```python
from build123d import *

# Parameters (mm, degrees)
F1_DEPTH    = 20
F0_W        = 58.4
F0_H        = 38.4
F2_DEPTH    = 75
F3_T1_DEPTH = 26
F4_R        = 8
F5_W        = 22
F5_H        = 6
F6_DEPTH    = 3


# Not quite as in the source:
# - a fillet or chamfer that OpenCascade refuses, or shapes differently, is made with other operations: its cross-section is extruded or revolved along the edge and cut away or added


with BuildPart() as f1:
    # F0 (on Top) → F1 (new body)
    with BuildSketch(Plane.XY):
        Polygon((20, -35.6130205363), (20, -33.6130205363), (-20, -33.6130205363), (-20, -35.6130205363), (-10, -35.6130205363), (10, -35.6130205363), align=None)
    extrude(amount=F1_DEPTH)

    # F0 (on Top) → F2 (join)
    with BuildSketch(Plane.XY):
        Polygon((20, -33.6130205363), (30, -33.6130205363), (30, 6.3869794637), (-30, 6.3869794637), (-30, -33.6130205363), (-20, -33.6130205363), align=None)
        with Locations((0, -13.6130205363)):
            Rectangle(F0_W, F0_H, mode=Mode.SUBTRACT)
    extrude(amount=F2_DEPTH)

    # F3: fillet of radius 1.2 on 4 edges, made by hand

    # F3_s2 → F3_t1 (cut)
    with BuildSketch(Plane.XY.offset(-3)):
        with BuildLine():
            ThreePointArc((20, -34.4130205363), (19.6485281374, -35.2615486737), (18.8, -35.6130205363))
            Line((18.8, -35.6130205363), (20, -35.6130205363))
            Line((20, -35.6130205363), (20, -34.4130205363))
        make_face()
        with BuildLine():
            ThreePointArc((-20, -34.4130205363), (-19.6485281374, -35.2615486737), (-18.8, -35.6130205363))
            Line((-18.8, -35.6130205363), (-20, -35.6130205363))
            Line((-20, -35.6130205363), (-20, -34.4130205363))
        make_face()
    extrude(amount=F3_T1_DEPTH, mode=Mode.SUBTRACT)

    # F4
    f4_edges = [f1.edges().sort_by_distance(p)[0] for p in [
        (29.2, 5.586979, 37.5),
        (29.2, -32.813021, 37.5),
        (-29.2, -32.813021, 37.5),
        (-29.2, 5.586979, 37.5),
        (-30, -33.613021, 37.5),
        (-30, 6.386979, 37.5),
        (30, -33.613021, 37.5),
        (30, 6.386979, 37.5),
    ]]
    fillet(f4_edges, radius=F4_R)

    # F5 (on face) → F6 (cut)
    with BuildSketch(Plane.XZ.offset(35.6130205363)):
        with Locations((0, 15)):
            Rectangle(F5_W, F5_H)
        with Locations((0, 6)):
            Rectangle(F5_W, F5_H)
    extrude(amount=-F6_DEPTH, mode=Mode.SUBTRACT)


solid = f1.part
```
Work out the finished part from the listing and answer in its coordinate system (mm). A direction names the side the tool comes from. Round coordinates to 2 decimals unless told otherwise and drop trailing zeros. Loops run counter-clockwise (first coordinate to the right, second up) from the corner with the lowest first, then second, coordinate; pieces in that order, holes last. Notation, with made-up numbers: (-35, -1.5) -> (-5, -1.5) arc R19 cw to (-5, 9.5) -> close; hole circle Ø10 at (33, 73.25). An arc over 180 degrees is marked (long way). Write each question's results on one line, items separated by ' | '. Start each with the question number.
1. Given pin 1 Ø1 at (x, y) = (4.5, -35) entering from +Z; pin 2 Ø1.4 at (y, z) = (-34.5, 5) entering from +X; pin 3 Ø1.4 at (y, z) = (-33.5, 6.5) entering from -X, each flat-ended and moving along its own axis, determine where each tip first touches the part or whether it passes through.
2. Find the intervals of material crossed by probe 1 along X at (y, z) = (-18, 31); probe 2 along Y at (x, z) = (7.5, 38); probe 3 along Y at (x, z) = (-9.5, 11.5), in increasing order. Write a range as from..to.
3. Section B-B (z = 36) is taken. Determine the outline of the cut face in (x, y), plus the area to 3 significant figures.
4. For a pull along Z with two mould halves and no side action, classify faces 1 (the face through (27.719, -31.207, 38.025)), 2 (the face through (0, -33, 0)), 3 (the face through (0, -34, 18)), 4 (the face through (11, -34, 6)) as +Z half, -Z half, draft (parallel to the pull), parting line (faces both ways), or undercut.
5. Section C-C (y = -11.5) is taken. Determine the outline of the cut face in (x, z).
6. Section A-A (x = 5.5) is taken. Determine the outline of the cut face in (y, z).
7. A tool of negligible diameter and unlimited length cuts with its end or side. For faces 5 (the face through (-11, -34, 15)), 6 (the face through (0, 5.587, 37)), 7 (the face through (-27.594, -31.332, 38.025)), from which of +Z, -Z, +X, -X, +Y, -Y can it reach the whole face along a straight path? Write none if from no direction.
8. Section D-D (x = 13) is taken. Determine the outline of the cut face in (y, z), plus the area to 3 significant figures.
Evaluation:
1) pin 1: stops at z = 20 | pin 2: stops at x = 20 | pin 3: stops at x = -25.51
2) probe 1: x = -30..-29.2, 29.2..30 | probe 2: y = -33.61..-32.81, 5.59..6.39 | probe 3: y = -35.61..-32.81, 5.59..6.39
3) outline: (-30, -25.61) arc R8 ccw to (-22, -33.61) -> (22, -33.61) arc R8 ccw to (30, -25.61) -> (30, -1.61) arc R8 ccw to (22, 6.39) -> (-22, 6.39) arc R8 ccw to (-30, -1.61) -> close; hole (-29.2, -24.81) arc R8 ccw to (-21.2, -32.81) -> (21.2, -32.81) arc R8 ccw to (29.2, -24.81) -> (29.2, -2.41) arc R8 ccw to (21.2, 5.59) -> (-21.2, 5.59) arc R8 ccw to (-29.2, -2.41) -> close | area: 157 mm2
4) face 1: draft | face 2: -Z half | face 3: undercut | face 4: undercut
5) outline: (-30, 0) -> (-29.2, 0) -> (-29.2, 75) -> (-30, 75) -> close; (29.2, 0) -> (30, 0) -> (30, 75) -> (29.2, 75) -> close
6) outline: (-35.61, 0) -> (-32.81, 0) -> (-32.81, 3) -> (-35.61, 3) -> close; (-35.61, 9) -> (-32.81, 9) -> (-32.81, 12) -> (-35.61, 12) -> close; (-35.61, 18) -> (-32.81, 18) -> (-32.81, 75) -> (-33.61, 75) -> (-33.61, 20) -> (-35.61, 20) -> close; (5.59, 0) -> (6.39, 0) -> (6.39, 75) -> (5.59, 75) -> close
7) face 5: -Y | face 6: +Z, -Z | face 7: +Z, -Z, -X, -Y
8) outline: (-35.61, 0) -> (-32.81, 0) -> (-32.81, 75) -> (-33.61, 75) -> (-33.61, 20) -> (-35.61, 20) -> close; (5.59, 0) -> (6.39, 0) -> (6.39, 75) -> (5.59, 75) -> close | area: 160 mm2
